Verification items for the finished model (mm, model axes). Face numbers are marked on the shaded views. A direction names the side the tool comes from. Round coordinates to 2 decimals unless told otherwise and drop trailing zeros. Order: outer loops, then holes, each group sorted by start corner. A loop starts at its lowest first (then second) coordinate and runs counter-clockwise, first axis right, second up. Notation, with made-up numbers: (-7, 26) -> (9, 26) arc R19 cw to (9, 58) -> close; hole circle Ø8 at (17, 37.25). An arc over 180 degrees is marked (long way). Put each result on its own line as item: value.
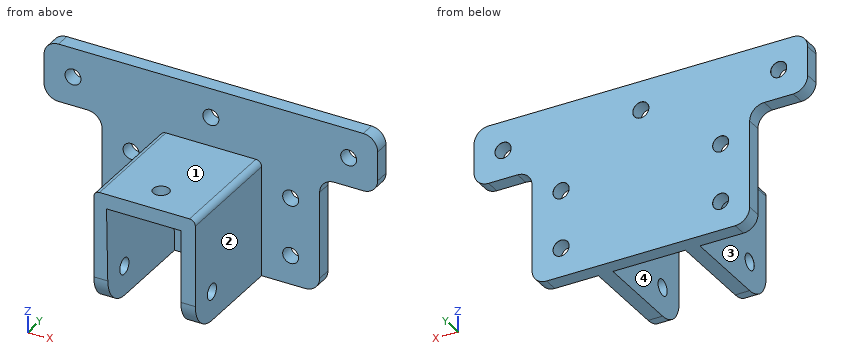
```python
from build123d import *

# Parameters (mm, degrees)
BOSS_EXTRUDE1_DEPTH            = 5
BOSS_EXTRUDE2_DEPTH            = 40
M5_CLEARANCE_HOLE1_D           = 5.5
M5_CLEARANCE_HOLE1_CSINK_D     = 5.55
M5_CLEARANCE_HOLE1_CSINK_ANGLE = 90
M5_CLEARANCE_HOLE2_D           = 5.5
M5_CLEARANCE_HOLE2_CSINK_D     = 5.55
M5_CLEARANCE_HOLE2_CSINK_ANGLE = 90
FILLET1_R                      = 2
M5_CLEARANCE_HOLE3_D           = 5.5
M5_CLEARANCE_HOLE3_CSINK_D     = 5.55
M5_CLEARANCE_HOLE3_CSINK_ANGLE = 90
FILLET2_R                      = 5
M5_CLEARANCE_HOLE4_D           = 5.5
M5_CLEARANCE_HOLE4_CSINK_D     = 5.55
M5_CLEARANCE_HOLE4_CSINK_ANGLE = 90
M5_CLEARANCE_HOLE5_D           = 5.5
M5_CLEARANCE_HOLE5_CSINK_D     = 5.55
M5_CLEARANCE_HOLE5_CSINK_ANGLE = 90
FILLET3_R                      = 10


with BuildPart() as part:
    # Sketch2 → Boss-Extrude1 (new body)
    with BuildSketch(Plane(origin=(0, 0, 0), x_dir=(1, 0, 0), z_dir=(0, 1, 0))):
        Polygon((-57.5, 0), (57.5, 0), (57.5, 20), (37.5, 20), (37.5, 60), (-37.5, 60), (-37.5, 20), (-57.5, 20), align=None)
    extrude(amount=BOSS_EXTRUDE1_DEPTH)

    # Sketch3 → Boss-Extrude2 (add)
    with BuildSketch(Plane.XZ):
        Polygon((17.5, -60), (17.5, -20), (-17.5, -20), (-17.5, -60), (-12.5, -60), (-13.096167181, -25), (12.5, -25), (12.5, -60), align=None)
    extrude(amount=BOSS_EXTRUDE2_DEPTH)

    # M5 Clearance Hole1 (through all)
    with Locations(Plane(origin=(-27.5, 5, -50), x_dir=(0, 0, 1), z_dir=(0, 1, 0))):
        with Locations((0, 0), (20, 0)):
            m5_clearance_hole1 = CounterSinkHole(M5_CLEARANCE_HOLE1_D / 2, M5_CLEARANCE_HOLE1_CSINK_D / 2, counter_sink_angle=M5_CLEARANCE_HOLE1_CSINK_ANGLE)

    # Mirror1: M5 Clearance Hole1 across plane
    add(m5_clearance_hole1.mirror(Plane(origin=(0, 0, 0), x_dir=(0, 0, 1), z_dir=(1, 0, 0))), mode=Mode.SUBTRACT)

    # M5 Clearance Hole2 (through all)
    with Locations(Plane(origin=(-47.5, 5, -10), x_dir=(0, 0, 1), z_dir=(0, 1, 0))):
        with Locations((0, 0)):
            m5_clearance_hole2 = CounterSinkHole(M5_CLEARANCE_HOLE2_D / 2, M5_CLEARANCE_HOLE2_CSINK_D / 2, counter_sink_angle=M5_CLEARANCE_HOLE2_CSINK_ANGLE)

    # Mirror2: M5 Clearance Hole2 across plane
    add(m5_clearance_hole2.mirror(Plane(origin=(0, 0, 0), x_dir=(0, 0, 1), z_dir=(1, 0, 0))), mode=Mode.SUBTRACT)

    # Fillet1
    fillet1_edges = [part.edges().sort_by_distance(p)[0] for p in [
        (17.5, -20, -20),
        (-17.5, -20, -20),
    ]]
    fillet(fillet1_edges, radius=FILLET1_R)

    # M5 Clearance Hole3 (through all)
    with Locations(Plane(origin=(0, -30, -25), x_dir=(-1, 0, 0), z_dir=(0, 0, -1))):
        with Locations((0, 0)):
            CounterSinkHole(M5_CLEARANCE_HOLE3_D / 2, M5_CLEARANCE_HOLE3_CSINK_D / 2, counter_sink_angle=M5_CLEARANCE_HOLE3_CSINK_ANGLE)

    # Fillet2
    fillet2_edges = [part.edges().sort_by_distance(p)[0] for p in [
        (37.5, 2.5, -20),
        (57.5, 2.5, -20),
        (57.5, 2.5, 0),
        (-57.5, 2.5, 0),
        (-57.5, 2.5, -20),
        (-37.5, 2.5, -20),
        (-37.5, 2.5, -60),
        (37.5, 2.5, -60),
    ]]
    fillet(fillet2_edges, radius=FILLET2_R)

    # M5 Clearance Hole4 (through all)
    with Locations(Plane(origin=(0, 5, -10), x_dir=(0, 0, 1), z_dir=(0, 1, 0))):
        with Locations((0, 0)):
            CounterSinkHole(M5_CLEARANCE_HOLE4_D / 2, M5_CLEARANCE_HOLE4_CSINK_D / 2, counter_sink_angle=M5_CLEARANCE_HOLE4_CSINK_ANGLE)

    # M5 Clearance Hole5 (through all)
    with Locations(Plane(origin=(-17.5, -30, -50), x_dir=(0, 0, -1), z_dir=(-1, 0, 0))):
        with Locations((0, 0)):
            CounterSinkHole(M5_CLEARANCE_HOLE5_D / 2, M5_CLEARANCE_HOLE5_CSINK_D / 2, counter_sink_angle=M5_CLEARANCE_HOLE5_CSINK_ANGLE)

    # Fillet3
    fillet3_edges = [part.edges().sort_by_distance(p)[0] for p in [
        (15, -40, -60),
        (-15, -40, -60),
    ]]
    fillet(fillet3_edges, radius=FILLET3_R)


solid = part.part
```
Item 1: Depth check by flat-ended pin: pin 1 Ø13 at (x, z) = (-1, -46) entering from -Y; pin 2 Ø4 at (y, z) = (-15, -35) entering from -X; pin 3 Ø1.5 at (y, z) = (-3.5, -35.5) entering from +X. Enter the tip coordinate at first touch or a pass-through.
Geometry check:
pin 1: y = 0
pin 2: x = -17.5
pin 3: x = 17.5
Item 2: Material ranges on line 1 along Z through (x, y) = (-27.5, 1.95); line 2 along X through (y, z) = (1, -10); line 3 along X through (y, z) = (2.8, -50), recorded low to high.
Geometry check:
line 1: -60 to -52.75, -47.25 to -32.75, -27.25 to 0
line 2: -57.5 to -50.25, -44.75 to -2.75, 2.75 to 44.75, 50.25 to 57.5
line 3: -37.5 to -30.25, -24.75 to 24.75, 30.25 to 37.5
Item 3: Sectioned sample at C-C, the plane x = -7. Record the boundary of the cut face in (y, z).
Geometry check:
outline: (-40, -25) -> (0, -25) -> (0, -60) -> (5, -60) -> (5, 0) -> (0, 0) -> (0, -20) -> (-40, -20) -> close
Item 4: Tool access check on the marked faces 1, 2, 3 and 4. Record the directions out of +Z, -Z, +X, -X, +Y, -Y that give a thin tool (end or side, any length) a straight path to the whole face; none if there is none.
Geometry check:
face 1: +Z, +X, -X, -Y
face 2: +Z, -Z, +X, -Y
face 3: +Z, -Z, -X, -Y
face 4: -Z, -Y
Item 5: Sectioned sample at B-B, the plane z = -10. Record the boundary of the cut face in (x, y) (3 decimals), then the cut area to 3 significant figures.
Geometry check:
outline: (-57.5, 0) -> (-50.25, 0) -> (-50.25, 4.975) -> (-50.275, 5) -> (-57.5, 5) -> close; (-44.75, 0) -> (-2.75, 0) -> (-2.75, 4.975) -> (-2.775, 5) -> (-44.725, 5) -> (-44.75, 4.975) -> close; (2.75, 0) -> (44.75, 0) -> (44.75, 4.975) -> (44.725, 5) -> (2.775, 5) -> (2.75, 4.975) -> close; (50.25, 0) -> (57.5, 0) -> (57.5, 5) -> (50.275, 5) -> (50.25, 4.975) -> close
area: 492 mm2
Item 6: Sectioned sample at D-D, the plane y = -18. Record the boundary of the cut face in (x, z), then the cut area to 3 significant figures.
Geometry check:
outline: (-17.5, -60) -> (-12.5, -60) -> (-13.1, -25) -> (12.5, -25) -> (12.5, -60) -> (17.5, -60) -> (17.5, -22) arc R2 ccw to (15.5, -20) -> (-15.5, -20) arc R2 ccw to (-17.5, -22) -> close
area: 513 mm2
Item 7: Sectioned sample at A-A, the plane x = -27.5. Record the boundary of the cut face in (y, z) (3 decimals), then the cut area to 3 significant figures.
Geometry check:
outline: (0, -60) -> (5, -60) -> (5, -52.775) -> (4.975, -52.75) -> (0, -52.75) -> close; (0, -47.25) -> (4.975, -47.25) -> (5, -47.225) -> (5, -32.775) -> (4.975, -32.75) -> (0, -32.75) -> close; (0, -27.25) -> (4.975, -27.25) -> (5, -27.225) -> (5, 0) -> (0, 0) -> close
area: 245 mm2
